Autodesk Fusion 360 part; units mm, degrees
sketch "Sketch1" plane through (0, 0, 0) normal (0, 1, 0) x (1, 0, 0)
  line L0 (0, 0) -> (0, -100)
  circle A0 centre (4.1857, -107.4765) radius 8.5685
  line L1 (4.1857, -1.3614) -> (4.1857, -1.2953)
  line L2 (8.3714, 0) -> (8.3714, -100)
  arc A1 (8.3714, 0) -> (0, 0) centre (4.1857, 6.1156) ccw
  dimension "d1" = 100
extrude "Extrude1" add sketch "Sketch1" along normal blind 5
sketch "Sketch2" plane through (0, 0, 0) normal (0, -1, 0) x (1, 0, 0)
  arc A0 (0, 0) -> (8.3714, 0) centre (4.1857, -6.1156) ccw
  line L0 (8.3714, 0) -> (8.3714, 100)
  arc A1 (8.3714, 100) -> (0, 100) centre (4.1857, 107.4765) ccw
  line L1 (0, 100) -> (0, 0)
  line L2 (3.0876, -2.0175) -> (1.1857, -0.9195)
  line L3 (7.1857, -0.9195) -> (5.2838, -2.0175)
  line L4 (0.0876, -5.0175) -> (-1.8143, -6.1156)
  line L5 (1.1857, -3.1156) -> (-1.0104, -3.1156)
  line L6 (4.1857, -0.1156) -> (3.0876, -2.0175)
  line L7 (0.0876, -7.2137) -> (-1.0104, -9.1156)
  line L8 (1.1857, -0.9195) -> (1.1857, -3.1156)
  line L9 (1.1857, -9.1156) -> (1.1857, -11.3118)
  line L10 (-1.0104, -3.1156) -> (0.0876, -5.0175)
  line L11 (3.0876, -10.2137) -> (4.1857, -12.1156)
  line L12 (-1.8143, -6.1156) -> (0.0876, -7.2137)
  line L13 (5.2838, -10.2137) -> (7.1857, -11.3118)
  line L14 (-1.0104, -9.1156) -> (1.1857, -9.1156)
  line L15 (7.1857, -9.1156) -> (9.3819, -9.1156)
  line L16 (1.1857, -11.3118) -> (3.0876, -10.2137)
  line L17 (8.2838, -7.2137) -> (10.1857, -6.1156)
  line L18 (4.1857, -12.1156) -> (5.2838, -10.2137)
  line L19 (8.2838, -5.0175) -> (9.3819, -3.1156)
  line L20 (7.1857, -11.3118) -> (7.1857, -9.1156)
  line L21 (7.1857, -3.1156) -> (7.1857, -0.9195)
  line L22 (9.3819, -9.1156) -> (8.2838, -7.2137)
  line L23 (5.2838, -2.0175) -> (4.1857, -0.1156)
  line L24 (10.1857, -6.1156) -> (8.2838, -5.0175)
  line L25 (9.3819, -3.1156) -> (7.1857, -3.1156)
  circle A2 centre (4.1857, 107.4765) radius 8.5685
  line L26 (-3.2037, 111.8142) -> (1.4127, 104.4395)
  line L27 (4.1857, 116.045) -> (8.8021, 108.6703)
  spline S0 degree 2 poles (8.8021, 108.6703) (6.4939, 104.4395) (1.4127, 104.4395) knots 0 0 0 0.931949 0.931949 0.931949 weights 1 3 1
  point P0 (4.1857, -6.1156)
  point P1 (4.1857, -6.1156)
  point P2 (4.1857, -6.1156)
  point P3 (4.1857, -6.1156)
  dimension "d5" = 6
  dimension "d6" = 6
  dimension "d7" = 6
  dimension "d8" = 6
extrude "Extrude2" cut sketch "Sketch2" along normal mid plane 18 contours A1 A2 L26 L27 S0 | L2 L3 L4 L5 L6 L7 L8 L9 L10 L11 L12 L13 L14 L15 L16 L17 L18 L19 L20 L21 L22 L23 L24 L25 picked at (4.1836, 108.8223)
sketch "Sketch3" plane through (0, 0, 0) normal (0, -1, 0) x (1, 0, 0)
  line L0 (1.4127, 104.4395) -> (-3.2037, 111.8142)
  arc A0 (-3.2037, 111.8142) -> (0, 100) centre (4.1857, 107.4765) ccw
  line L1 (0, 100) -> (0, 0)
  arc A1 (0, 0) -> (8.3714, 0) centre (4.1857, -6.1156) ccw
  line L2 (8.3714, 0) -> (8.3714, 100)
  arc A2 (8.3714, 100) -> (4.1857, 116.045) centre (4.1857, 107.4765) ccw
  line L3 (4.1857, 116.045) -> (8.8021, 108.6703)
  spline S0 degree 3 poles (8.8021, 108.6703) (7.7372, 106.7184) (7.1677, 105.8398) (6.3827, 105.0938) (6.1105, 104.9214) (5.074, 104.5294) (3.9773, 104.4395) (1.4127, 104.4395) knots 0 0 0 0 0.667054 0.667054 1.004366 1.004366 1.733719 1.733719 1.733719 1.733719
  line L4 (7.1857, -0.9195) -> (7.1857, -3.1156)
  line L5 (7.1857, -3.1156) -> (9.3819, -3.1156)
  line L6 (9.3819, -3.1156) -> (8.2838, -5.0175)
  line L7 (8.2838, -5.0175) -> (10.1857, -6.1156)
  line L8 (10.1857, -6.1156) -> (8.2838, -7.2137)
  line L9 (8.2838, -7.2137) -> (9.3819, -9.1156)
  line L10 (9.3819, -9.1156) -> (7.1857, -9.1156)
  line L11 (7.1857, -9.1156) -> (7.1857, -11.3118)
  line L12 (7.1857, -11.3118) -> (5.2838, -10.2137)
  line L13 (5.2838, -10.2137) -> (4.1857, -12.1156)
  line L14 (4.1857, -12.1156) -> (3.0876, -10.2137)
  line L15 (3.0876, -10.2137) -> (1.1857, -11.3118)
  line L16 (1.1857, -11.3118) -> (1.1857, -9.1156)
  line L17 (1.1857, -9.1156) -> (-1.0104, -9.1156)
  line L18 (-1.0104, -9.1156) -> (0.0876, -7.2137)
  line L19 (0.0876, -7.2137) -> (-1.8143, -6.1156)
  line L20 (-1.8143, -6.1156) -> (0.0876, -5.0175)
  line L21 (0.0876, -5.0175) -> (-1.0104, -3.1156)
  line L22 (-1.0104, -3.1156) -> (1.1857, -3.1156)
  line L23 (1.1857, -3.1156) -> (1.1857, -0.9195)
  line L24 (1.1857, -0.9195) -> (3.0876, -2.0175)
  line L25 (3.0876, -2.0175) -> (4.1857, -0.1156)
  line L26 (4.1857, -0.1156) -> (5.2838, -2.0175)
  line L27 (5.2838, -2.0175) -> (7.1857, -0.9195)
  line L28 (1.6279, 96.2747) -> (1.6245, 4.7564)
  arc A3 (1.6245, 4.7564) -> (6.7471, 4.7562) centre (4.1858, 4.7563) ccw
  line L29 (6.7471, 4.7562) -> (6.7504, 96.2745)
  arc A4 (6.7504, 96.2745) -> (1.6279, 96.2747) centre (4.1891, 96.2746) ccw
  line L30 (4.1892, 98.8359) -> (4.1857, 2.195) construction
extrude "Extrude3" cut sketch "Sketch3" against normal blind 1 contours L28 A3 L29 A4
extrude "Extrude4" cut 1 faces at (4.1857, 5, 66.6281) along direction (0, -1, 0) blind 1
Verification items for the finished model (mm, model axes). A direction names the side the tool comes from. Coordinates: 2 decimals unless noted, no trailing zeros. Loops run counter-clockwise (first coordinate to the right, second up) from the corner with the lowest first, then second, coordinate; pieces in that order, holes last. Notation, with made-up numbers: (61, -32) - (112, -32) arc R9 cw to (112, -27) - close; hole circle Ø5 at (27.25, 18). An arc over 180 degrees is marked (long way). Return JSON: item names as keys, results as strings.
1. Mould release check, pull along X, two halves, no side actions. Record for faces 5 (the cylindrical face through (-4.1, 2, 105.3)), 6 (the cylindrical face through (4.246, 0.493, 98.835)), 7 (the cylindrical face through (12.515, 1.972, 109.486)), 8 (the flat face through (4, 4, 50)): +X half, -X half, draft (parallel to the pull), parting line (faces both ways), or undercut.
Established:
{"face 5": "-X half", "face 6": "undercut", "face 7": "+X half", "face 8": "draft"}
2. Go/stop test with flat-tipped pins: pin 1 (1.8 mm diameter, centred on y = 1.5, z = -10, fed in from -X); pin 2 (1.1 mm diameter, centred on x = 8.5, y = 2.5, fed in from +Z); pin 3 (0.8 mm diameter, centred on y = 0.5, z = 58.5, fed in from +X); pin 4 (2 mm diameter, centred on x = -2.5, z = 31, fed in from -Y). Record where each tip stops, or that it passes through.
Established:
{"pin 1": "stops at x = -2.6", "pin 2": "stops at z = 115.17", "pin 3": "stops at x = 8.37", "pin 4": "passes through"}
3. Tool access check on faces 1 (the flat face through (4, 1, 51)), 2 (the flat face through (0, 2, 49)), 3 (the flat face through (6.46, 1.97, 112.41)), 4 (the flat face through (-0.93, 1.97, 108.18)). Record the directions out of +Z, -Z, +X, -X, +Y, -Y that give a thin tool (end or side, any length) a straight path to the whole face; none if there is none.
Established:
{"face 1": "-Y", "face 2": "-X, +Y, -Y", "face 3": "+Y, -Y", "face 4": "+Z, +Y, -Y"}
4. Thickness scan on L1, parallel to X at y = 0.2, z = 26; L2, parallel to Z at x = 2.5, y = 0.45; L3, parallel to Z at x = 2, y = 0.9. Record the ranges inside material, lowest first.
Established:
{"L1": "x = 0 to 1.63, 6.75 to 8.37", "L2": "z = -13.33 to -10.55, -1.68 to 2.83, 98.2 to 104.45", "L3": "z = -13.2 to -10.84, -1.39 to 3.42, 97.6 to 104.44"}
5. Section check A-A, the plane z = 67. Record the boundary of the cut face in (x, y), then the cut area to 3 significant figures.
Established:
{"outline": "(0, 0) - (1.63, 0) - (1.63, 1) - (6.75, 1) - (6.75, 0) - (8.37, 0) - (8.37, 4) - (0, 4) - close", "area": "28.4 mm2"}
